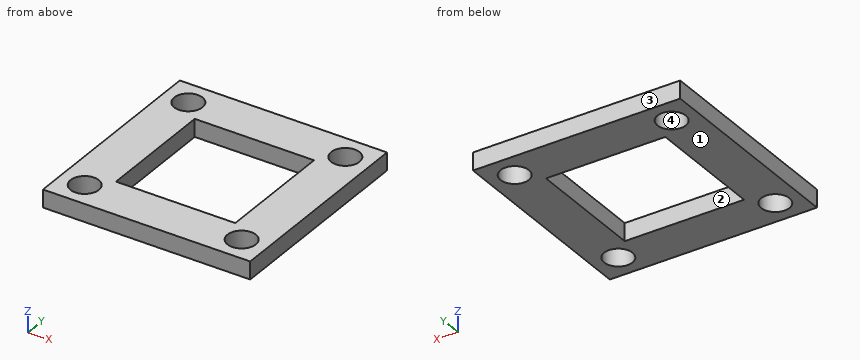
from build123d import *

# Parameters (mm, degrees)
SKETCH1_W           = 23.33452378
SKETCH1_H           = 23.33452378
SKETCH1_W_2         = 13.435028842
SKETCH1_H_2         = 13.435028842
BOSS_EXTRUDE1_DEPTH = 1
SKETCH2_R           = 1.6
CUT_EXTRUDE1_DEPTH  = 3


with BuildPart() as part:
    # Sketch1 → Boss-Extrude1 (new body, symmetric)
    with BuildSketch(Plane.XY):
        Rectangle(SKETCH1_W, SKETCH1_H)
        Rectangle(SKETCH1_W_2, SKETCH1_H_2, mode=Mode.SUBTRACT)
    extrude(amount=BOSS_EXTRUDE1_DEPTH, both=True)

    # Sketch2 → Cut-Extrude1 (cut, through all)
    with BuildSketch(Plane(origin=(0, 0, -1), x_dir=(-1, 0, 0), z_dir=(0, 0, -1))):
        with Locations((8.838834765, -8.838834765)):
            Circle(SKETCH2_R)
        with Locations((8.838834765, 8.838834765)):
            Circle(SKETCH2_R)
        with Locations((-8.838834765, -8.838834765)):
            Circle(SKETCH2_R)
        with Locations((-8.838834765, 8.838834765)):
            Circle(SKETCH2_R)
    extrude(amount=-CUT_EXTRUDE1_DEPTH, mode=Mode.SUBTRACT)


solid = part.part
Build history of the part. All positions in model axes, mm. Face numbers are marked on the shaded views. A direction names the side the tool comes from. Coordinates: 2 decimals unless noted, no trailing zeros. Order: outer loops, then holes, each group sorted by start corner. A loop starts at its lowest first (then second) coordinate and runs counter-clockwise, first axis right, second up. Notation, with made-up numbers: M -13.75,67 L 0.25,67 A18 ccw 0.25,78 Z; hole C 3.25,85.5 d11. An arc over 180 degrees is marked long. One line per question, with ' | ' between items. Start each with the question number.
Q1. Saw through at D-D (x = -10). List the corners of the cut face in (y, z), then the cut area to 3 significant figures.
Q2. Probe L1, parallel to X at y = -4.25, z = 0.75; L2, parallel to X at y = 9.75, z = 0.8. List the from-to ranges inside material, lowest first. Write a range as from..to.
Q3. Saw through at C-C (z = 0.4). List the corners of the cut face in (x, y).
Q4. Two-plate mould, pull along X, no slides. Class the marked faces 3 and 4: +X half, -X half, draft (parallel to the pull), parting line (faces both ways), or undercut.
Q5. Flat gauge pin, fed straight in: pin 1 Ø1.9 at (x, y) = (8.84, -8.84) entering from +Z. Where does the tip first touch, or does it go through?
Q6. Saw through at A-A (y = 0.5). List the corners of the cut face in (x, z), then the cut area to 3 significant figures.
Q7. 3-axis set-ups, long thin cutter, end or side, ignore diameter. For the marked faces 1 and 2: which of +Z, -Z, +X, -X, +Y, -Y reach the whole face in a straight line?
Check values:
1) outline: M -11.67,-1 L -9.94,-1 L -9.94,1 L -11.67,1 Z; M -7.74,-1 L 7.74,-1 L 7.74,1 L -7.74,1 Z; M 9.94,-1 L 11.67,-1 L 11.67,1 L 9.94,1 Z | area: 37.9 mm2
2) L1: x = -11.67..-6.72, 6.72..11.67 | L2: x = -11.67..-10.15, -7.52..7.52, 10.15..11.67
3) outline: M -11.67,-11.67 L 11.67,-11.67 L 11.67,11.67 L -11.67,11.67 Z; hole C -8.84,-8.84 d3.2; hole C -8.84,8.84 d3.2; hole M -6.72,-6.72 L 6.72,-6.72 L 6.72,6.72 L -6.72,6.72 Z; hole C 8.84,-8.84 d3.2; hole C 8.84,8.84 d3.2
4) face 3: draft | face 4: undercut
5) pin 1: passes through
6) outline: M -11.67,-1 L -6.72,-1 L -6.72,1 L -11.67,1 Z; M 6.72,-1 L 11.67,-1 L 11.67,1 L 6.72,1 Z | area: 19.8 mm2
7) face 1: -Z, +X, -X, +Y, -Y | face 2: +Z, -Z
